from build123d import *

# Parameters (mm, degrees)
SKETCH1_W           = 43.699940619
SKETCH1_H           = 33.102984907
BOSS_EXTRUDE1_DEPTH = 10
BOSS_EXTRUDE3_DEPTH = 10
M5_TAPPED_HOLE1_D   = 4.2
SKETCH18_W          = 13
SKETCH18_H          = 47.102984907
CUT_EXTRUDE1_DEPTH  = 10
SKETCH20_W          = 10
SKETCH20_H          = 17.102984907
CUT_EXTRUDE3_DEPTH  = 10
SKETCH22_W          = 20.699940619
SKETCH22_H          = 17.102984907
BOSS_EXTRUDE4_DEPTH = 17.3288
SKETCH23_W          = 58.662437665
SKETCH23_H          = 17.102984907
BOSS_EXTRUDE5_DEPTH = 10
BOSS_EXTRUDE6_DEPTH = 20
M8_TAPPED_HOLE3_D   = 6.8
FILLET4_R           = 5
FILLET6_R           = 5
FILLET7_R           = 1


with BuildPart() as part:
    # Sketch1 → Boss-Extrude1 (new body)
    with BuildSketch(Plane.XY):
        Polygon((42.979890311, 22.079670103), (-49.382487973, 22.079670103), (-49.382487973, -7.920329897), (-5.682547354, -7.920329897), (42.979890311, -7.920329897), align=None)
        with Locations((-27.532517664, -24.471822351)):
            Rectangle(SKETCH1_W, SKETCH1_H)
    extrude(amount=BOSS_EXTRUDE1_DEPTH)

    # Sketch10 → Boss-Extrude3 (add, symmetric)
    with BuildSketch(Plane(origin=(0, 7.079670103, 0), x_dir=(-1, 0, 0), z_dir=(0, -1, 0))):
        Polygon((-24.707127971, -10), (-24.707127971, -12.991563555), (-41.673127971, -10), align=None)
    extrude(amount=BOSS_EXTRUDE3_DEPTH, both=True)

    # M5 Tapped Hole1 (through all)
    with Locations(Plane(origin=(35.156022436, 6.992687386, 11.149141542), x_dir=(0.984807753012, 0, -0.173648177667), z_dir=(0.173648177667, 0, 0.984807753012))):
        with Locations((0, 0)):
            Hole(M5_TAPPED_HOLE1_D / 2)

    # Sketch18 → Cut-Extrude1 (cut)
    with BuildSketch(Plane.XY.offset(10)):
        Polygon((-36.382487973, -25.023314804), (-49.382487973, -25.023314804), (-49.382487973, -41.023314804), (-5.682547354, -41.023314804), (-5.682547354, -25.023314804), align=None)
        with Locations((-42.882487973, -1.471822351)):
            Rectangle(SKETCH18_W, SKETCH18_H)
    extrude(amount=-CUT_EXTRUDE1_DEPTH, mode=Mode.SUBTRACT)

    # Sketch20 → Cut-Extrude3 (cut)
    with BuildSketch(Plane(origin=(0, 0, 0), x_dir=(-1, 0, 0), z_dir=(0, 0, -1))):
        with Locations((10.682547354, -16.471822351)):
            Rectangle(SKETCH20_W, SKETCH20_H)
    extrude(amount=-CUT_EXTRUDE3_DEPTH, mode=Mode.SUBTRACT)

    # Sketch22 → Boss-Extrude4 (add)
    with BuildSketch(Plane.XY.offset(10)):
        with Locations((-26.032517664, -16.471822351)):
            Rectangle(SKETCH22_W, SKETCH22_H)
    extrude(amount=BOSS_EXTRUDE4_DEPTH)

    # Sketch23 → Boss-Extrude5 (add)
    with BuildSketch(Plane(origin=(0, 0, 0), x_dir=(-1, 0, 0), z_dir=(0, 0, -1))):
        with Locations((-13.648671479, -16.471822351)):
            Rectangle(SKETCH23_W, SKETCH23_H)
    extrude(amount=-BOSS_EXTRUDE5_DEPTH)

    # Sketch27 → Boss-Extrude6 (add)
    with BuildSketch(Plane.XY.offset(27.3288)):
        with BuildLine():
            Line((-36.382487973, -25.023314804), (-15.730623406, -25.023314804))
            ThreePointArc((-15.730623406, -25.023314804), (-12.1950895, -23.55884871), (-10.730623406, -20.023314804))
            Line((-10.730623406, -20.023314804), (-10.730623406, -4.371450237))
            ThreePointArc((-10.730623406, -4.371450237), (-12.1950895, -0.835916331), (-15.730623406, 0.628549763))
            Line((-15.730623406, 0.628549763), (-31.382487973, 0.628549763))
            ThreePointArc((-31.382487973, 0.628549763), (-34.918021878, -0.835916331), (-36.382487973, -4.371450237))
            Line((-36.382487973, -4.371450237), (-36.382487973, -25.023314804))
        make_face()
    extrude(amount=-BOSS_EXTRUDE6_DEPTH)

    # M8 Tapped Hole3 (through all)
    with Locations(Plane(origin=(-28.692487973, -14.540329897, 0), x_dir=(-1, 0, 0), z_dir=(0, 0, -1))):
        with Locations((0, 0)):
            Hole(M8_TAPPED_HOLE3_D / 2)

    # Fillet4
    fillet4_edges = [part.edges().sort_by_distance(p)[0] for p in [
        (-36.382487973, -25.023314804, 13.6644),
    ]]
    fillet(fillet4_edges, radius=FILLET4_R)

    # Fillet6
    fillet6_edges = [part.edges().sort_by_distance(p)[0] for p in [
        (-36.382487973, 22.079670103, 5),
        (42.979890311, 22.079670103, 5),
        (42.979890311, -25.023314804, 5),
    ]]
    fillet(fillet6_edges, radius=FILLET6_R)

    # Fillet7
    fillet7_edges = [part.edges().sort_by_distance(p)[0] for p in [
        (3.298701169, -25.023314804, 0),
        (-34.918021878, -23.55884871, 0),
        (3.298701169, 22.079670103, 0),
        (-36.382487973, -1.471822351, 0),
        (42.979890311, -1.471822351, 0),
        (-34.918021878, 20.615204009, 0),
        (41.515424217, -23.55884871, 0),
        (41.515424217, 20.615204009, 0),
    ]]
    fillet(fillet7_edges, radius=FILLET7_R)


solid = part.part
Here's how the part is built. I have some questions about the finished solid (model axes, mm). A direction names the side the tool comes from. Round coordinates to 2 decimals unless told otherwise and drop trailing zeros. Order: outer loops, then holes, each group sorted by start corner. A loop starts at its lowest first (then second) coordinate and runs counter-clockwise, first axis right, second up. Notation, with made-up numbers: M 2.5,69 L 18.5,69 A25 ccw 18.5,95 Z; hole C 28.25,-21.75 d4. An arc over 180 degrees is marked long. Return JSON: item names as keys, results as strings. Group by question number.
1. If we section it at C-C on x = -24: List the corners of the cut face in (y, z) for me, then the cut area to 3 significant figures.
2. If we mould it in two halves opening along X, with no side actions, what happens to faces 4 (the face through (24.707, 7, 11)), 5 (the face through (31.19, 6.94, 11.85)), 6 (the face through (-25.55, -15.84, 13.86)), 7 (the face through (-23, 0.629, 19))? For each: pulls with the +X half, pulls with the -X half, needs draft (parallel to the pull), parting line crosses it, or undercut.
3. If we section it at D-D on y = -6.5: List the corners of the cut face in (x, z) for me.
4. On a 3-axis mill with a long thin cutter (end or side, diameter ignored), from which of +Z, -Z, +X, -X, +Y, -Y can I reach the whole of each face in a straight line? I mean faces 1 (the face through (-34.88, -0.8, 18.79)), 2 (the face through (4, 22.08, 5)), 3 (the face through (31, -2.92, 11)). Say none if no direction works.
5. I'm going to push flat-ended pins straight in: pin 1 Ø2.5 at (y, z) = (4.5, 11.5) entering from -X; pin 2 Ø5 at (x, y) = (29.5, -8) entering from +Z; pin 3 Ø8 at (y, z) = (-13, 17.5) entering from +X. Where does each tip first touch, or does it pass through?
6. If we section it at A-A on y = 10: List the corners of the cut face in (x, z) for me, then the cut area to 3 significant figures.
7. Please list where these lines run through material, in increasing order: probe 1 along Z at (x, y) = (-8.5, 11.5); probe 2 along X at (y, z) = (-17, 16.5); probe 3 along X at (y, z) = (-13.5, 14).
Reply:
{
 "1": {"outline": "M -25.02,1 A1 ccw -24.02,0 L 21.08,0 A1 ccw 22.08,1 L 22.08,10 L 0.63,10 L 0.63,27.33 L -25.02,27.33 Z", "area": "915 mm^2"},
 "2": {"face 4": "undercut", "face 5": "pulls with the +X half", "face 6": "undercut", "face 7": "needs draft"},
 "3": {"outline": "M -36.38,1 A1 ccw -35.38,0 L 41.98,0 A1 ccw 42.98,1 L 42.98,10 L -10.73,10 L -10.73,27.33 L -36.38,27.33 Z"},
 "4": {"face 1": "+Z, -X, +Y", "face 2": "+Z, -Z, +X, -X, +Y", "face 3": "+Z, +X, -Y"},
 "5": {"pin 1": "x = 24.71", "pin 2": "z = 10", "pin 3": "x = -10.73"},
 "6": {"outline": "M -36.38,1 A1 ccw -35.38,0 L 41.98,0 A1 ccw 42.98,1 L 42.98,10 L 41.67,10 L 24.71,12.99 L 24.71,10 L -36.38,10 Z", "area": "819 mm^2"},
 "7": {"probe 1": "0 to 10", "probe 2": "-36.38 to -31.04, -26.35 to -10.73", "probe 3": "-36.38 to -31.93, -25.46 to -10.73"}
}
